```python
from build123d import *

# Parameters (mm, degrees)
SKETCH001_R       = 0.9
PAD001_DEPTH      = 10.67
PAD001_DEPTH_BACK = 3.5
SKETCH_R          = 13.95
SKETCH_R_2        = 1.46
PAD_DEPTH         = 21.34
FILLET_R          = 0.5


with BuildPart() as pad001:
    # Sketch001 → Pad001 (new body, two sides)
    with BuildSketch(Plane.XY.offset(0.5)) as pad001_sk:
        Circle(SKETCH001_R)
        with Locations((20.07, 0)):
            Circle(SKETCH001_R)
    extrude(amount=PAD001_DEPTH)
    extrude(pad001_sk.sketch, amount=-PAD001_DEPTH_BACK)


with BuildPart() as obj1:
    # Sketch → Pad (new body)
    with BuildSketch(Plane.XY.offset(0.1)):
        with Locations((10.035, 0)):
            Circle(SKETCH_R)
        with Locations((10.035, 0)):
            Circle(SKETCH_R_2, mode=Mode.SUBTRACT)
    extrude(amount=PAD_DEPTH)

    # Fillet
    fillet_edges = [obj1.edges().sort_by_distance(p)[0] for p in [
        (8.575, 0, 21.44),
        (-3.915, 0, 21.44),
        (-3.915, 0, 0.1),
    ]]
    fillet(fillet_edges, radius=FILLET_R)

    # obj1: union Pad001
    add(pad001.part)


solid = obj1.part
```
Verification items for the finished model (mm, model axes). A direction names the side the tool comes from. Give positions to 0.01 mm unless a question says otherwise; leave off trailing zeros. Write each loop counter-clockwise with the first axis right and the second up, starting at its lowest first coordinate (ties: lowest second). Pieces come first, ordered by that corner, then holes. Notation, with made-up numbers: (4, 73.25) - (51, 73.25) arc R5 ccw to (51, 77.25) - close; hole circle Ø9 at (24.25, 32.5). An arc over 180 degrees is marked (long way). Put each result on its own line as item: value.
Q1. Mould release check, pull along X, two halves, no side actions. Record for faces 3 (the face through (0, 0, -3)), 4 (the face through (8.576, 0.064, 10.374)), 5 (the face through (0.86, 0.27, -1.43)), 6 (the face through (23.34, 4.19, 10.63)): released by +X, released by -X, zero draft, split by the parting line, or undercut.
Result:
face 3: zero draft
face 4: undercut
face 5: undercut
face 6: split by the parting line
Q2. Set-up check for faces 1 (the face through (10, -3, 21.44)), 2 (the face through (19.17, 0.04, -1.43)): record each of +Z, -Z, +X, -X, +Y, -Y from which the full face is reachable in a straight line by a thin tool's end or side.
Result:
face 1: +Z, +X, -X, +Y, -Y
face 2: -Z
Q3. Section check A-A on y = 0. Record the cut outline in (x, z) (3 decimals).
Result:
outline: (-3.915, 0.6) arc R0.5 ccw to (-3.415, 0.1) - (-0.9, 0.1) - (-0.9, -3) - (0.9, -3) - (0.9, 0.1) - (8.575, 0.1) - (8.575, 20.94) arc R0.5 ccw to (8.075, 21.44) - (-3.415, 21.44) arc R0.5 ccw to (-3.915, 20.94) - close; (11.495, 0.1) - (19.17, 0.1) - (19.17, -3) - (20.97, -3) - (20.97, 0.1) - (23.485, 0.1) arc R0.5 ccw to (23.985, 0.6) - (23.985, 20.94) arc R0.5 ccw to (23.485, 21.44) - (11.995, 21.44) arc R0.5 ccw to (11.495, 20.94) - close
Q4. Scan lines: probe 1 along Y at (x, z) = (10, 8.5); probe 2 along Z at (x, y) = (21, 1.75); probe 3 along Y at (x, z) = (11.25, 4). Record each from-to range of solid material in increasing order. Write a range as from..to.
Result:
probe 1: -13.95..-1.46, 1.46..13.95
probe 2: 0.1..21.44
probe 3: -13.9..-0.81, 0.81..13.9
Q5. Section check B-B on z = 7.5. Record the cut outline in (x, y) (3 decimals), and give its area (3 significant figures).
Result:
outline: circle Ø27.9 at (10.035, 0); hole circle Ø2.92 at (10.035, 0)
area: 605 mm2
Q6. Depth check by flat-ended pin: P1, Ø5, axis at x = 14, y = 10.5, coming from the -Z side; P2, Ø1.5, axis at x = 16, z = 3, coming from the -Y side; P3, Ø13.5, axis at x = 7, y = -2.5, coming from the -Z side; P4, Ø2.5, axis at x = 10.035, y = 0, coming from the -Z side. Enter the tip coordinate at first touch or a pass-through.
Result:
P1: z = 0.1
P2: y = -12.94
P3: z = -3
P4: through
